The listing builds one solid part. Answer for the finished solid, in the listing's coordinates (mm). A direction names the side the tool comes from. Give positions to 0.01 mm unless a question says otherwise; leave off trailing zeros. Write each loop counter-clockwise with the first axis right and the second up, starting at its lowest first coordinate (ties: lowest second). Pieces come first, ordered by that corner, then holes. Notation, with made-up numbers: (61, 80) -> (118, 80) arc R6 cw to (118, 86) -> close; hole circle Ø10 at (61, 29). An arc over 180 degrees is marked (long way). Put each result on its own line as item: value. Start each with the question number.
1) A cutting plane is placed at C-C (z = 5.5). Write down the section's boundary in (x, y).
2) Find the intervals of material crossed by line 1 along Y through (x, z) = (0, 2.5); line 2 along X through (y, z) = (-3, 6.5); line 3 along Z through (x, y) = (-3.5, -14), in increasing order. Write a range as from..to.
3) Flat-ended cylindrical pins translate along their axes: pin 1 Ø10.5 at (x, y) = (0, 0) entering from +Z; pin 2 Ø5 at (y, z) = (-16.5, 5) entering from +X; pin 3 Ø2 at (y, z) = (-8, 5) entering from +X. Find the tip coordinate at first contact, or state that the pin passes through.
4) A cutting plane is placed at A-A (y = 0). Write down the section's boundary in (x, z).
5) For a pull along X with two mould halves and no side action, classify faces 3 (the cylindrical face through (-0.759, 8.583, 3.451)), 4 (the cylindrical face through (13.17, 20.66, 4.45)), 5 (the flat face through (0, -5, 0)) as released by +X, released by -X, zero draft, split by the parting line, or undercut.
6) For faces 1 (the flat face through (3, -3, 7)), 2 (the cylindrical face through (8.503, 0.154, 3.451)), determine the directions among +Z, -Z, +X, -X, +Y, -Y from which every point of the face is accessible in a straight line to the end or side of a thin tool.
from build123d import *

# Parameters (mm, degrees)
SKETCH1_R           = 24.5
SKETCH1_R_2         = 18
BOSS_EXTRUDE1_DEPTH = 9
SKETCH1_3_R         = 18
SKETCH1_3_R_2       = 16
SKETCH1_3_R_3       = 4
SKETCH1_3_R_4       = 3.5
BOSS_EXTRUDE2_DEPTH = 7


with BuildPart() as part:
    # Sketch1 → Boss-Extrude1 (new body)
    with BuildSketch(Plane.XY):
        Circle(SKETCH1_R)
        Circle(SKETCH1_R_2, mode=Mode.SUBTRACT)
    extrude(amount=BOSS_EXTRUDE1_DEPTH)

    # Sketch1_3 → Boss-Extrude2 (add)
    # profile 1 of 2: a face of its own
    with BuildSketch(Plane.XY):
        Circle(SKETCH1_3_R)
        Circle(SKETCH1_3_R_2, mode=Mode.SUBTRACT)
    # profile 2 of 2: a face of its own
    with BuildSketch(Plane.XY):
        Circle(SKETCH1_3_R_2)
        Circle(SKETCH1_3_R_3, mode=Mode.SUBTRACT)
        with Locations((-12, 0)):
            Circle(SKETCH1_3_R_4, mode=Mode.SUBTRACT)
        with Locations((0, -12)):
            Circle(SKETCH1_3_R_4, mode=Mode.SUBTRACT)
        with Locations((12, 0)):
            Circle(SKETCH1_3_R_4, mode=Mode.SUBTRACT)
        with Locations((0, 12)):
            Circle(SKETCH1_3_R_4, mode=Mode.SUBTRACT)
    extrude(amount=BOSS_EXTRUDE2_DEPTH)

    # Sketch3 → Revolve2 (revolve)
    with BuildSketch(Plane(origin=(0, 0, 0), x_dir=(1, 0, 0), z_dir=(0, 1, 0)), mode=Mode.PRIVATE) as revolve2_sk:
        Polygon((-18, -9), (-16, -7), (-18, -7), align=None)
    revolve(revolve2_sk.sketch.rotate(Axis((0, 0, -3.771799992), (0, 0, 1)), 180), axis=Axis((0, 0, -3.771799992), (0, 0, 1)))

    # Sketch4 → Cut-Revolve1 (revolve, cut)
    with BuildSketch(Plane(origin=(0, 0, 0), x_dir=(1, 0, 0), z_dir=(0, 1, 0))):
        Polygon((-24.5, -8), (-23.5, -9), (-24.5, -9), align=None)
        Polygon((-24.5, -1), (-23.5, 0), (-24.5, 0), align=None)
    revolve(axis=Axis((0, 0, -7.551154296), (0, 0, 1)), mode=Mode.SUBTRACT)


solid = part.part
Reply:
1. outline: circle Ø49 at (0, 0); hole circle Ø7 at (-12, 0); hole circle Ø8 at (0, 0); hole circle Ø7 at (0, -12); hole circle Ø7 at (0, 12); hole circle Ø7 at (12, 0)
2. line 1: y = -24.5..-15.5, -8.5..-4, 4..8.5, 15.5..24.5
2. line 2: x = -24.32..-13.8, -10.2..-2.65, 2.65..10.2, 13.8..24.32
2. line 3: z = 0..7
3. pin 1: stops at z = 7
3. pin 2: stops at x = 20.11
3. pin 3: stops at x = 23.48
4. outline: (-24.5, 1) -> (-23.5, 0) -> (-15.5, 0) -> (-15.5, 7) -> (-16, 7) -> (-18, 9) -> (-23.5, 9) -> (-24.5, 8) -> close; (-8.5, 0) -> (-4, 0) -> (-4, 7) -> (-8.5, 7) -> close; (4, 0) -> (8.5, 0) -> (8.5, 7) -> (4, 7) -> close; (15.5, 0) -> (23.5, 0) -> (24.5, 1) -> (24.5, 8) -> (23.5, 9) -> (18, 9) -> (16, 7) -> (15.5, 7) -> close
5. face 3: undercut
5. face 4: split by the parting line
5. face 5: zero draft
6. face 1: +Z
6. face 2: +Z, -Z
